CAD build for the part. Positions are in the model's coordinates, mm. A direction names the side the tool comes from. Coordinates: 2 decimals unless noted, no trailing zeros. Write each loop counter-clockwise with the first axis right and the second up, starting at its lowest first coordinate (ties: lowest second). Pieces come first, ordered by that corner, then holes. Notation, with made-up numbers: (26.5, 36.5) - (82.5, 36.5) arc R24 cw to (82.5, 71.5) - close; hole circle Ø10 at (13, -33). An arc over 180 degrees is marked (long way). Answer in a Markdown table with one row per item. Add a question column.
Q1. Band-saw the part on B-B (z = -12). List the corners of the cut face in (x, y) (3 decimals), and give its area (3 significant figures).
Q2. Drill centre lines: line 1 along X through (y, z) = (-7.5, -25.4) (3 decimals); line 2 along Z through (x, y) = (-48, -6) (3 decimals); line 3 along X through (y, z) = (-13, -25.4) (3 decimals). Where is each one in solid material? Low to high. Write a range as from..to.
Q3. 3-axis set-ups, long thin cutter, end or side, ignore diameter. For faces 1 (the flat face through (43, -3.175, 1)), 2 (the flat face through (0, -12.7, 1)), 3 (the flat face through (43, -15.875, 1)): which of +Z, -Z, +X, -X, +Y, -Y reach the whole face in a straight line?
Q4. Band-saw the part on A-A (y = -8.25). List the corners of the cut face in (x, z) (3 decimals), and give its area (3 significant figures).
Q5. Band-saw the part on D-D (y = -1.25). List the corners of the cut face in (x, z), and give its area (3 significant figures).
Q6. Pin check, flat tips, straight feed: pin 1 (2.5 mm diameter, centred on y = -1.5, z = 9.5, fed in from +X); pin 2 (8 mm diameter, centred on x = 5.5, z = -21, fed in from -Y); pin 3 (1 mm diameter, centred on y = -2.5, z = -14.5, fed in from -X); pin 4 (8 mm diameter, centred on x = -47.625, z = 25.4, fed in from -Y) (3 decimals). Stop position of each tip, or through.
Q7. Band-saw the part on C-C (x = -18). List the corners of the cut face in (y, z).
Q8. Two-plate mould, pull along X, no slides. Class faces 4 (the flat face through (1, -8, -38.1)), 5 (the flat face through (-25.4, -14, 1)), 6 (the cylindrical face through (-56.506, -9.436, 34.478)), 7 (the cylindrical face through (-45.599, -10.234, 26.953)): +X half, -X half, draft (parallel to the pull), parting line (faces both ways), or undercut.
```python
from build123d import *

# Parameters (mm, degrees)
BOSS_EXTRUDE1_DEPTH               = 38.1
FILLET1_R                         = 12.7
F_1_4_20_TAPPED_HOLE1_D           = 5.1054
F_1_4_20_TAPPED_HOLE1_CSINK_D     = 7.62
F_1_4_20_TAPPED_HOLE1_CSINK_ANGLE = 90


with BuildPart() as part:
    # Sketch1 → Boss-Extrude1 (new, symmetric)
    with BuildSketch(Plane.XY):
        Polygon((-25.4, 0), (25.4, 0), (25.4, -3.175), (60.325, -3.175), (60.325, -15.875), (25.4, -15.875), (25.4, -12.7), (-25.4, -12.7), (-25.4, -15.875), (-60.325, -15.875), (-60.325, -3.175), (-25.4, -3.175), align=None)
    extrude(amount=BOSS_EXTRUDE1_DEPTH, both=True)

    # Fillet1
    fillet1_edges = [part.edges().sort_by_distance(p)[0] for p in [
        (-60.325, -9.525, 38.1),
        (60.325, -9.525, -38.1),
        (-60.325, -9.525, -38.1),
        (60.325, -9.525, 38.1),
    ]]
    fillet(fillet1_edges, radius=FILLET1_R)

    # 1/4-20 Tapped Hole1 (through all)
    with Locations(Plane(origin=(0, -3.175, 0), x_dir=(1, 0, 0), z_dir=(0, 1, 0))):
        with Locations((-47.625, 25.4), (-47.625, -25.4), (47.625, -25.4), (47.625, 25.4)):
            CounterSinkHole(F_1_4_20_TAPPED_HOLE1_D / 2, F_1_4_20_TAPPED_HOLE1_CSINK_D / 2, counter_sink_angle=F_1_4_20_TAPPED_HOLE1_CSINK_ANGLE)


solid = part.part
```
Checked values:
| question | item | result |
|---|---|---|
| 1 | outline | (-60.325, -15.875) - (-25.4, -15.875) - (-25.4, -12.7) - (25.4, -12.7) - (25.4, -15.875) - (60.325, -15.875) - (60.325, -3.175) - (25.4, -3.175) - (25.4, 0) - (-25.4, 0) - (-25.4, -3.175) - (-60.325, -3.175) - close |
| 1 | area | 1,530 mm² |
| 2 | line 1 | x = -60.325..-50.178, -45.072..45.072, 50.178..60.325 |
| 2 | line 2 | z = -38.094..-27.925, -22.875..22.875, 27.925..38.094 |
| 2 | line 3 | x = -60.325..-50.178, -45.072..-25.4, 25.4..45.072, 50.178..60.325 |
| 3 | face 1 | +Z, -Z, +X, +Y |
| 3 | face 2 | +Z, -Z, -Y |
| 3 | face 3 | +Z, -Z, +X, -X, -Y |
| 4 | outline | (-60.325, -25.4) arc R12.7 ccw to (-47.625, -38.1) - (47.625, -38.1) arc R12.7 ccw to (60.325, -25.4) - (60.325, 25.4) arc R12.7 ccw to (47.625, 38.1) - (-47.625, 38.1) arc R12.7 ccw to (-60.325, 25.4) - close; hole circle Ø5.105 at (-47.625, -25.4); hole circle Ø5.105 at (-47.625, 25.4); hole circle Ø5.105 at (47.625, -25.4); hole circle Ø5.105 at (47.625, 25.4) |
| 4 | area | 8,970 mm² |
| 5 | outline | (-25.4, -38.1) - (25.4, -38.1) - (25.4, 38.1) - (-25.4, 38.1) - close |
| 5 | area | 3,870 mm² |
| 6 | pin 1 | stops at x = 25.4 |
| 6 | pin 2 | stops at y = -12.7 |
| 6 | pin 3 | stops at x = -25.4 |
| 6 | pin 4 | stops at y = -15.875 |
| 7 | outline | (-12.7, -38.1) - (0, -38.1) - (0, 38.1) - (-12.7, 38.1) - close |
| 8 | face 4 | draft |
| 8 | face 5 | undercut |
| 8 | face 6 | -X half |
| 8 | face 7 | undercut |
